Source: CAD feature listing. Evaluate the final solid. Frame: model axes, mm. Face numbers are marked on the shaded views. A direction names the side the tool comes from. Round coordinates to 2 decimals unless told otherwise and drop trailing zeros. Loops run counter-clockwise (first coordinate to the right, second up) from the corner with the lowest first, then second, coordinate; pieces in that order, holes last. Notation, with made-up numbers: M 10,29.5 L 41,29.5 A17 cw 41,55.5 Z; hole C 70.5,61.5 d1. An arc over 180 degrees is marked long. Answer as a JSON object with one key per item and string values.
from build123d import *

# Parameters (mm, degrees)
F1_DEPTH = 7.8
F2_START = 0.8
F0_R     = 2.4
F2_DEPTH = 6.2
F0_R_2   = 1
F0_R_3   = 2
F3_DEPTH = 0.8


# Not quite as in the source:
# - a feature names something its author has since deleted; it is built from what else it names


with BuildPart() as f1:
    # F0 (on Top) → F1 (new body)
    with BuildSketch(Plane.XY):
        with BuildLine():
            ThreePointArc((0, 11.7), (-2.6162950904, 10.6162950904), (-3.7, 8))
            Line((-3.7, 8), (-3.7, 7.7))
            ThreePointArc((-3.7, 7.7), (-3.9928932188, 6.9928932188), (-4.7, 6.7))
            Line((-4.7, 6.7), (-6.1, 6.7))
            ThreePointArc((-6.1, 6.7), (-7.2313708499, 6.2313708499), (-7.7, 5.1))
            Line((-7.7, 5.1), (-7.7, -5.1))
            ThreePointArc((-7.7, -5.1), (-7.2313708499, -6.2313708499), (-6.1, -6.7))
            Line((-6.1, -6.7), (-4.7, -6.7))
            ThreePointArc((-4.7, -6.7), (-3.9928932188, -6.9928932188), (-3.7, -7.7))
            Line((-3.7, -7.7), (-3.7, -8))
            ThreePointArc((-3.7, -8), (-2.6162950904, -10.6162950904), (0, -11.7))
            ThreePointArc((0, -11.7), (2.6162950904, -10.6162950904), (3.7, -8))
            Line((3.7, -8), (3.7, -7.7))
            ThreePointArc((3.7, -7.7), (3.9928932188, -6.9928932188), (4.7, -6.7))
            Line((4.7, -6.7), (6.1, -6.7))
            ThreePointArc((6.1, -6.7), (7.2313708499, -6.2313708499), (7.7, -5.1))
            Line((7.7, -5.1), (7.7, 5.1))
            ThreePointArc((7.7, 5.1), (7.2313708499, 6.2313708499), (6.1, 6.7))
            Line((6.1, 6.7), (4.7, 6.7))
            ThreePointArc((4.7, 6.7), (3.9928932188, 6.9928932188), (3.7, 7.7))
            Line((3.7, 7.7), (3.7, 8))
            ThreePointArc((3.7, 8), (2.6162950904, 10.6162950904), (0, 11.7))
        make_face()
        with BuildLine():
            Line((-6.1, -5.1), (-6.1, 5.1))
            Line((-6.1, 5.1), (-1.3527749258, 5.1))
            ThreePointArc((-1.3527749258, 5.1), (-1.7191742549, 10.698970152), (3.2, 8))
            ThreePointArc((3.2, 8), (2.698970152, 6.2808257451), (1.3527749258, 5.1))
            Line((1.3527749258, 5.1), (6.1, 5.1))
            Line((6.1, 5.1), (6.1, -5.1))
            Line((6.1, -5.1), (1.3527749258, -5.1))
            ThreePointArc((1.3527749258, -5.1), (2.698970152, -6.2808257451), (3.2, -8))
            ThreePointArc((3.2, -8), (-1.7191742549, -10.698970152), (-1.3527749258, -5.1))
            Line((-1.3527749258, -5.1), (-6.1, -5.1))
        make_face(mode=Mode.SUBTRACT)
    extrude(amount=F1_DEPTH)

    # F0 (on Top) → F2 (join)
    with BuildSketch(Plane.XY.offset(F2_START)):
        with BuildLine():
            Line((1.3527749258, -5.1), (-1.3527749258, -5.1))
            ThreePointArc((-1.3527749258, -5.1), (-1.7191742549, -10.698970152), (3.2, -8))
            ThreePointArc((3.2, -8), (2.698970152, -6.2808257451), (1.3527749258, -5.1))
        make_face()
        with Locations((0, -8)):
            Circle(F0_R, mode=Mode.SUBTRACT)
        with BuildLine():
            ThreePointArc((3.2, 8), (-1.7191742549, 10.698970152), (-1.3527749258, 5.1))
            Line((-1.3527749258, 5.1), (1.3527749258, 5.1))
            ThreePointArc((1.3527749258, 5.1), (2.698970152, 6.2808257451), (3.2, 8))
        make_face()
        with Locations((0, 8)):
            Circle(F0_R, mode=Mode.SUBTRACT)
    extrude(amount=F2_DEPTH)

    # F0 (on Top) → F3 (join)
    with BuildSketch(Plane.XY):
        with BuildLine():
            Line((-1.3527749258, 5.1), (-6.1, 5.1))
            Line((-6.1, 5.1), (-6.1, -5.1))
            Line((-6.1, -5.1), (-1.3527749258, -5.1))
            ThreePointArc((-1.3527749258, -5.1), (0, -4.8), (1.3527749258, -5.1))
            Line((1.3527749258, -5.1), (6.1, -5.1))
            Line((6.1, -5.1), (6.1, 5.1))
            Line((6.1, 5.1), (1.3527749258, 5.1))
            ThreePointArc((1.3527749258, 5.1), (0, 4.8), (-1.3527749258, 5.1))
        make_face()
        with Locations((-4.5, 0)):
            Circle(F0_R_2, mode=Mode.SUBTRACT)
        Circle(F0_R_3, mode=Mode.SUBTRACT)
        with Locations((4.5, 0)):
            Circle(F0_R_2, mode=Mode.SUBTRACT)
    extrude(amount=F3_DEPTH)


solid = f1.part
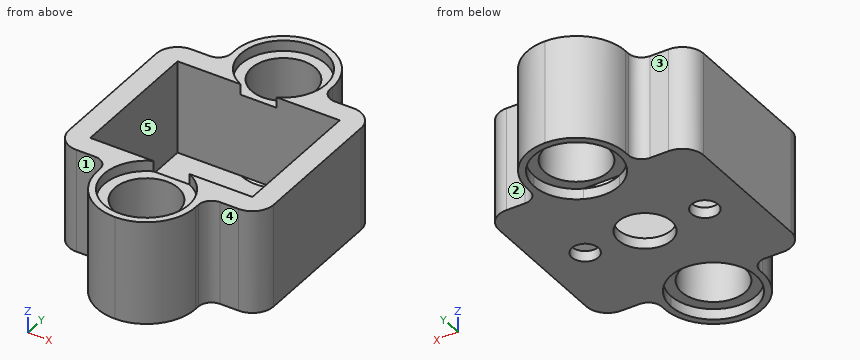
Item 1: Section B-B on y = 3.5. Return the cut outline in (x, z), then the cut area to 3 significant figures.
Answer sheet:
{"outline": "M -7.7,0 L 7.7,0 L 7.7,7.8 L 6.1,7.8 L 6.1,0.8 L -6.1,0.8 L -6.1,7.8 L -7.7,7.8 Z", "area": "34.7 mm²"}
Item 2: Access query for the marked faces 1, 2, 3, 4 and 5. Directions: +Z, -Z, +X, -X, +Y, -Y. A direction counts if a zero-diameter tool reaches every point of the face in a straight line with its end or side. Return the directions, or none.
Answer sheet:
{"face 1": "+Z, -Z, -X, -Y", "face 2": "+Z, -Z, +X, +Y", "face 3": "+Z, -Z, -X, +Y", "face 4": "+Z, -Z, +X, -Y", "face 5": "+Z"}
Item 3: Section D-D on y = 10. Return the cut outline in (x, z), then the cut area to 3 significant figures.
Answer sheet:
{"outline": "M -3.11,0 L -2.5,0 L -2.5,0.8 L -1.33,0.8 L -1.33,7 L -2.5,7 L -2.5,7.8 L -3.11,7.8 Z; M 1.33,0.8 L 2.5,0.8 L 2.5,0 L 3.11,0 L 3.11,7.8 L 2.5,7.8 L 2.5,7 L 1.33,7 Z", "area": "24.1 mm²"}
Item 4: Section C-C on z = 4. Return the cut outline in (x, y).
Answer sheet:
{"outline": "M -7.7,-5.1 A1.6 ccw -6.1,-6.7 L -4.7,-6.7 A1 cw -3.7,-7.7 L -3.7,-8 A3.7 ccw 3.7,-8 L 3.7,-7.7 A1 cw 4.7,-6.7 L 6.1,-6.7 A1.6 ccw 7.7,-5.1 L 7.7,5.1 A1.6 ccw 6.1,6.7 L 4.7,6.7 A1 cw 3.7,7.7 L 3.7,8 A3.7 ccw -3.7,8 L -3.7,7.7 A1 cw -4.7,6.7 L -6.1,6.7 A1.6 ccw -7.7,5.1 Z; hole M -6.1,-5.1 L 6.1,-5.1 L 6.1,5.1 L -6.1,5.1 Z; hole C 0,-8 d4.8; hole C 0,8 d4.8"}
Item 5: Section A-A on z = 7.25. Return the cut outline in (x, y).
Answer sheet:
{"outline": "M -7.7,-5.1 A1.6 ccw -6.1,-6.7 L -4.7,-6.7 A1 cw -3.7,-7.7 L -3.7,-8 A3.7 ccw 3.7,-8 L 3.7,-7.7 A1 cw 4.7,-6.7 L 6.1,-6.7 A1.6 ccw 7.7,-5.1 L 7.7,5.1 A1.6 ccw 6.1,6.7 L 4.7,6.7 A1 cw 3.7,7.7 L 3.7,8 A3.7 ccw -3.7,8 L -3.7,7.7 A1 cw -4.7,6.7 L -6.1,6.7 A1.6 ccw -7.7,5.1 Z; hole M -6.1,-5.1 L -1.35,-5.1 A3.2 ccw long 1.35,-5.1 L 6.1,-5.1 L 6.1,5.1 L 1.35,5.1 A3.2 ccw long -1.35,5.1 L -6.1,5.1 Z"}
Item 6: Contact query for flat-ended pins moving along their axis: pin 1 Ø8.5 at (x, y) = (0, -8) entering from -Z; pin 2 Ø3 at (x, y) = (-1.5, 7.5) entering from -Z; pin 3 Ø1.8 at (x, y) = (-4.5, 0) entering from +Z; pin 4 Ø1.5 at (y, z) = (-6.5, 2.5) entering from -X. Output: stop coordinate, or through.
Answer sheet:
{"pin 1": "stops at z = 0", "pin 2": "stops at z = 0.8", "pin 3": "passes through", "pin 4": "stops at x = -7.56"}
Item 7: Line query: probe 1 along Y at (x, z) = (0, 3.75); probe 2 along X at (y, z) = (3.25, 2.25); probe 3 along Y at (x, z) = (5.25, 2.5). Output: solid intervals per line, ascending. Write a range as from..to.
Answer sheet:
{"probe 1": "y = -11.7..-10.4, -5.6..-5.1, 5.1..5.6, 10.4..11.7", "probe 2": "x = -7.7..-6.1, 6.1..7.7", "probe 3": "y = -6.7..-5.1, 5.1..6.7"}
